Source: CAD feature listing. Evaluate the final solid. Frame: model axes, mm. A direction names the side the tool comes from. Round coordinates to 2 decimals unless told otherwise and drop trailing zeros. Write each loop counter-clockwise with the first axis right and the second up, starting at its lowest first coordinate (ties: lowest second). Pieces come first, ordered by that corner, then holes. Notation, with made-up numbers: M 6,64.25 L 64,64.25 A18 cw 64,83.25 Z; hole C -39.5,-11 d11. An arc over 180 degrees is marked long. Answer in a Markdown table with one row per item.
from build123d import *

# Parameters (mm, degrees)
BOSS_EXTRUDE1_DEPTH = 31.75
SKETCH2_R           = 2
CUT_EXTRUDE1_DEPTH  = 58.12585076
CUT_EXTRUDE2_REACH  = 62.42
SKETCH3_W           = 4.4
SKETCH3_H           = 2.771281292
CUT_EXTRUDE3_START  = -9
CUT_EXTRUDE3_DEPTH  = 9
CUT_EXTRUDE4_REACH  = 62.42
SKETCH5_R           = 2.5


with BuildPart() as part:
    # Sketch1 → Boss-Extrude1 (new body)
    with BuildSketch(Plane.XY):
        Polygon((-3.175, 0), (3.175, 0), (3.175, -38.1), (22.335, -38.1), (22.335, -34.29), (12.175, -34.29), (12.175, 3.81), (-12.175, 3.81), (-12.175, -34.29), (-22.335, -34.29), (-22.335, -38.1), (-3.175, -38.1), align=None)
    extrude(amount=BOSS_EXTRUDE1_DEPTH)

    # Sketch2 → Cut-Extrude1 (cut, through all)
    with BuildSketch(Plane.XZ.offset(38.1)):
        with Locations(Location((-16.51, 25.4, 0), (0, 0, 270))):
            Circle(SKETCH2_R)
        with Locations(Location((16.51, 25.4, 0), (0, 0, 270))):
            Circle(SKETCH2_R)
    extrude(amount=-CUT_EXTRUDE1_DEPTH, mode=Mode.SUBTRACT)

    # Sketch3 → Cut-Extrude2 (cut, up to next)
    with BuildSketch(Plane.ZY.offset(12.175), mode=Mode.PRIVATE) as cut_extrude2_sk1:
        with Locations((6.35, -19.05)):
            Rectangle(SKETCH3_W, SKETCH3_H)
    cut_extrude2_tool1 = extrude(cut_extrude2_sk1.sketch, amount=-CUT_EXTRUDE2_REACH, mode=Mode.PRIVATE) & part.part
    add(cut_extrude2_tool1.solids().sort_by_distance((-12.175, -19.05, 6.35))[0], mode=Mode.SUBTRACT)

    # Sketch4 → Cut-Extrude3 (cut)
    with BuildSketch(Plane.ZY.offset(12.175).offset(CUT_EXTRUDE3_START)):
        with BuildLine():
            Line((4.15, -20.435640646), (4.15, -17.664359354))
            ThreePointArc((4.15, -17.664359354), (6.35, -16.45), (8.55, -17.664359354))
            Line((8.55, -17.664359354), (8.55, -20.435640646))
            ThreePointArc((8.55, -20.435640646), (6.35, -21.65), (4.15, -20.435640646))
        make_face()
    extrude(amount=CUT_EXTRUDE3_DEPTH, mode=Mode.SUBTRACT)

    # Sketch5 → Cut-Extrude4 (cut, up to next)
    with BuildSketch(Plane(origin=(12.175, 0, 0), x_dir=(0, 0, -1), z_dir=(1, 0, 0)), mode=Mode.PRIVATE) as cut_extrude4_sk1:
        with Locations(Location((-6.35, -19.05, 0), (0, 0, 90))):
            Circle(SKETCH5_R)
    cut_extrude4_tool1 = extrude(cut_extrude4_sk1.sketch, amount=-CUT_EXTRUDE4_REACH, mode=Mode.PRIVATE) & part.part
    add(cut_extrude4_tool1.solids().sort_by_distance((12.175, -19.05, 6.35))[0], mode=Mode.SUBTRACT)


solid = part.part
Q1. Contact query for flat-ended pins moving along their axis: pin 1 Ø1 at (y, z) = (-3, 21.5) entering from +X (3 decimals); pin 2 Ø9.5 at (y, z) = (-7.5, 15) entering from -X (3 decimals); pin 3 Ø4.5 at (y, z) = (-19.05, 6.35) entering from +X (3 decimals). Output: stop coordinate, or through.
Solutions:
| item | result |
|---|---|
| pin 1 | stops at x = 12.175 |
| pin 2 | stops at x = -12.175 |
| pin 3 | stops at x = -3.175 |
Q2. Section C-C (z = 6.35). Return loops of the section in (x, y) (3 decimals).
Solutions:
| item | result |
|---|---|
| outline | M -22.335,-38.1 L -3.175,-38.1 L -3.175,-21.65 L -12.175,-21.65 L -12.175,-34.29 L -22.335,-34.29 Z; M -12.175,-16.45 L -3.175,-16.45 L -3.175,0 L 3.175,0 L 3.175,-16.55 L 12.175,-16.55 L 12.175,3.81 L -12.175,3.81 Z; M 3.175,-38.1 L 22.335,-38.1 L 22.335,-34.29 L 12.175,-34.29 L 12.175,-21.55 L 3.175,-21.55 Z |
Q3. Access query for faces 1 (the cylindrical face through (-7.61, -21.65, 6.39)), 2 (the flat face through (-12.175, -15, 16)), 3 (the flat face through (12.175, -16, 16)), 4 (the cylindrical face through (7.74, -19.38, 8.83)). Directions: +Z, -Z, +X, -X, +Y, -Y. A direction counts if a zero-diameter tool reaches every point of the face in a straight line with its end or side. Return the directions, or none.
Solutions:
| item | result |
|---|---|
| face 1 | -X |
| face 2 | +Z, -Z, -X, +Y |
| face 3 | +Z, -Z, +X, +Y |
| face 4 | +X |
Q4. Section B-B (x = 16.51). Return loops of the section in (y, z).
Solutions:
| item | result |
|---|---|
| outline | M -38.1,0 L -34.29,0 L -34.29,23.4 L -38.1,23.4 Z; M -38.1,27.4 L -34.29,27.4 L -34.29,31.75 L -38.1,31.75 Z |
Q5. Section A-A (y = -4.5). Return loops of the section in (x, z) (3 decimals).
Solutions:
| item | result |
|---|---|
| outline | M -12.175,0 L -3.175,0 L -3.175,31.75 L -12.175,31.75 Z; M 3.175,0 L 12.175,0 L 12.175,31.75 L 3.175,31.75 Z |
Q6. Material intervals for probe 1 along X at (y, z) = (-17.5, 29) (3 decimals); probe 2 along X at (y, z) = (-34.5, 17) (3 decimals); probe 3 along Z at (x, y) = (-10, -18.5), sorted ascending.
Solutions:
| item | result |
|---|---|
| probe 1 | x = -12.175 to -3.175, 3.175 to 12.175 |
| probe 2 | x = -22.335 to -3.175, 3.175 to 22.335 |
| probe 3 | z = 0 to 4.15, 8.55 to 31.75 |
Q7. Pull-direction query (Y, two-part tool) for faces 5 (the flat face through (22.335, -36, 16)), 6 (the flat face through (13, -38.1, 16)), 7 (the flat face through (-8, -19, 8.55)); classes: pulls with the +Y half, pulls with the -Y half, needs draft (parallel to the pull), parting line crosses it, or undercut.
Solutions:
| item | result |
|---|---|
| face 5 | needs draft |
| face 6 | pulls with the -Y half |
| face 7 | undercut |
Q8. Section D-D (y = -18.5). Return loops of the section in (x, z) (3 decimals), and give its area (3 significant figures).
Solutions:
| item | result |
|---|---|
| outline | M -12.175,0 L -3.175,0 L -3.175,4.15 L -12.175,4.15 Z; M -12.175,8.55 L -3.175,8.55 L -3.175,31.75 L -12.175,31.75 Z; M 3.175,0 L 12.175,0 L 12.175,3.911 L 3.175,3.911 Z; M 3.175,8.789 L 12.175,8.789 L 12.175,31.75 L 3.175,31.75 Z |
| area | 488 mm2 |
